from build123d import *

# Parameters (mm, degrees)
EXTRUDE1_DEPTH              = 25.4
F_1_4_20_TAPPED_HOLE2_D     = 5.1054
F_1_4_20_TAPPED_HOLE2_DEPTH = 16.002
F_1_4_20_TAPPED_HOLE2_TIP   = 1.533816902


with BuildPart() as part:
    # Sketch1 → Extrude1 (new body)
    with BuildSketch(Plane.XY):
        Polygon((-8.815807595, 41.879239751), (-21.52120708, 25.279287896), (-21.52120708, -11.990787033), (-8.815807595, -11.990787033), align=None)
    extrude(amount=EXTRUDE1_DEPTH)

    # 1/4-20 Tapped Hole2
    with Locations(Plane(origin=(7.200348194, -11.990787033, 18.061260674), x_dir=(-1, 0, 0), z_dir=(0, -1, 0))):
        with Locations((22.929112651, 5.361260674)):
            Hole(F_1_4_20_TAPPED_HOLE2_D / 2, depth=F_1_4_20_TAPPED_HOLE2_DEPTH)
            with Locations((0, 0, -(F_1_4_20_TAPPED_HOLE2_DEPTH + F_1_4_20_TAPPED_HOLE2_TIP / 2))):  # 118° drill point
                Cone(0, F_1_4_20_TAPPED_HOLE2_D / 2, F_1_4_20_TAPPED_HOLE2_TIP, mode=Mode.SUBTRACT)


solid = part.part
Here's how the part is built. I have some questions about the finished solid (model axes, mm). A direction names the side the tool comes from. Coordinates: 2 decimals unless noted, no trailing zeros. Loops run counter-clockwise (first coordinate to the right, second up) from the corner with the lowest first, then second, coordinate; pieces in that order, holes last.
1. For P1, Ø6.5, axis at x = -15.73, z = 12.7, coming from the +Y side; P2, Ø2, axis at x = -19.5, z = 12, coming from the +Y side, each with a flat end and sliding along its axis, tell me the tip position at first contact or that it passes through.
2. Imagine slicing it at B-B, the plane z = 17.25. Please give me the cut outline in (x, y), and give its area (3 significant figures).
3. For faces 1 (the cylindrical face through (-16.282, -3.878, 15.192)), 2 (the flat face through (-21.521, 7, 13)), which set-ups out of +Z, -Z, +X, -X, +Y, -Y let a thin tool reach every point of the face, with its end or its side?
4. If we mould it in two halves opening along X, with no side actions, what happens to faces 3 (the flat face through (-15, 9, 25.4)), 4 (the conical face through (-15.67, 5.28, 12.26)), 5 (the flat face through (-8.816, 15, 13))? For each: pulls with the +X half, pulls with the -X half, needs draft (parallel to the pull), parting line crosses it, or undercut.
5. I need wall thicknesses on L1, parallel to X at y = -5.5, z = 12.7; L2, parallel to Y at x = -18.5, z = 4.25; L3, parallel to Y at x = -10, z = 19.5. Which ranges of each line are inside material? Lowest first, please.
6. Imagine slicing it at C-C, the plane x = -20. Please give me the cut outline in (y, z).
7. Imagine slicing it at A-A, the plane y = 4.5. Please give me the cut outline in (x, z).
Taken from the geometry:
1. P1: stops at y = 37.09
1. P2: stops at y = 29.23
2. outline: (-21.52, -11.99) - (-8.82, -11.99) - (-8.82, 41.88) - (-21.52, 25.28) - close
2. area: 579 mm2
3. face 1: -Y
3. face 2: +Z, -Z, -X, +Y, -Y
4. face 3: needs draft
4. face 4: undercut
4. face 5: pulls with the +X half
5. L1: x = -21.52 to -18.28, -13.18 to -8.82
5. L2: y = -11.99 to 29.23
5. L3: y = -11.99 to 40.33
6. outline: (-11.99, 0) - (27.27, 0) - (27.27, 25.4) - (-11.99, 25.4) - close
7. outline: (-21.52, 0) - (-8.82, 0) - (-8.82, 25.4) - (-21.52, 25.4) - close; hole circle Ø3.48 at (-15.73, 12.7)
